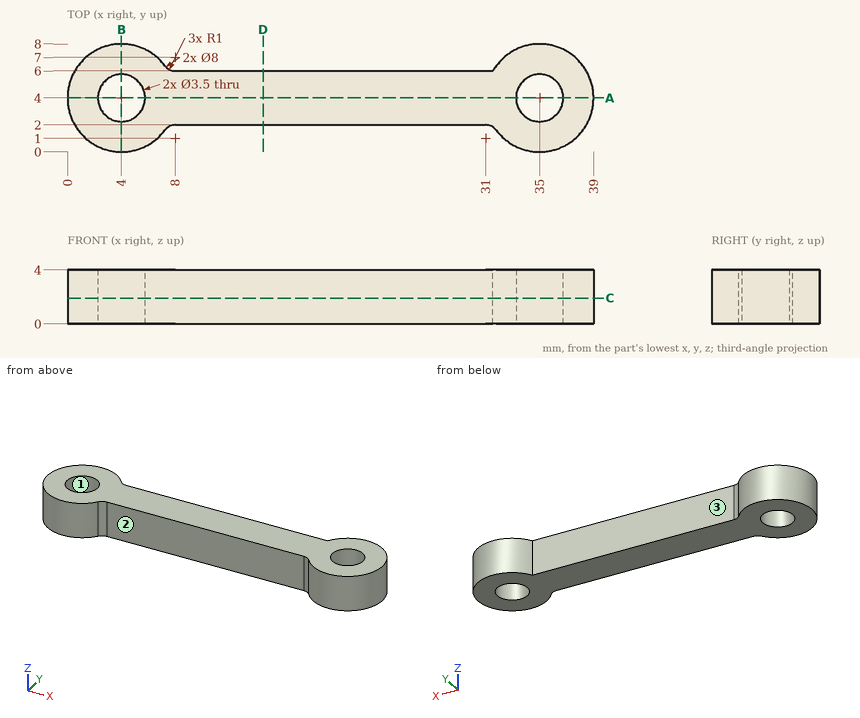
Answer from the drawing. Dimensions are ordinates in mm from the lowest x, y and z of the part. Coordinates: 2 decimals unless noted, no trailing zeros. Loops run counter-clockwise (first coordinate to the right, second up) from the corner with the lowest first, then second, coordinate; pieces in that order, holes last. Notation, with made-up numbers: (88.25, -5) - (138.25, -5) arc R11 cw to (138.25, 3) - close; hole circle Ø6 at (-34, 32). An arc over 180 degrees is marked (long way). Use a Markdown table: item, result.
Item 1: The mould has two halves that part along Y. Classify the marked faces 1, 2 and 3: +Y half, -Y half, draft (parallel to the pull), parting line (faces both ways), or undercut.
Evaluation:
| item | result |
|---|---|
| face 1 | undercut |
| face 2 | -Y half |
| face 3 | +Y half |
Item 2: Consider probe 1 along Y at (x, z) = (35, 1.9); probe 2 along X at (y, z) = (2.5, 3.15); probe 3 along X at (y, z) = (3.5, 3.85). Determine where each line is inside the solid, lowest interval first. Write a range as from..to.
Evaluation:
| item | result |
|---|---|
| probe 1 | y = 0..2.25, 5.75..8 |
| probe 2 | x = 0.29..3.1, 4.9..34.1, 35.9..38.71 |
| probe 3 | x = 0.03..2.32, 5.68..33.32, 36.68..38.97 |
Item 3: Find section A-A, the plane y = 4. Determine the outline of the cut face in (x, z).
Evaluation:
| item | result |
|---|---|
| outline | (0, 0) - (2.25, 0) - (2.25, 4) - (0, 4) - close; (5.75, 0) - (33.25, 0) - (33.25, 4) - (5.75, 4) - close; (36.75, 0) - (39, 0) - (39, 4) - (36.75, 4) - close |
Item 4: Find section B-B, the plane x = 4. Determine the outline of the cut face in (y, z), and give its area (3 significant figures).
Evaluation:
| item | result |
|---|---|
| outline | (0, 0) - (2.25, 0) - (2.25, 4) - (0, 4) - close; (5.75, 0) - (8, 0) - (8, 4) - (5.75, 4) - close |
| area | 18.0 mm2 |
Item 5: Given pin 1 Ø2 at (x, z) = (15, 1.5) entering from -Y; pin 2 Ø1.5 at (y, z) = (3, 3.5) entering from +X; pin 3 Ø3 at (x, y) = (13, 5.5) entering from -Z; pin 4 Ø1 at (y, z) = (1, 2.5) entering from -X, each flat-ended and moving along its own axis, determine where each tip first touches the part or whether it passes through.
Evaluation:
| item | result |
|---|---|
| pin 1 | stops at y = 2 |
| pin 2 | stops at x = 38.99 |
| pin 3 | stops at z = 0 |
| pin 4 | stops at x = 0.88 |
Item 6: Find section D-D, the plane x = 14.5. Determine the outline of the cut face in (y, z).
Evaluation:
| item | result |
|---|---|
| outline | (2, 0) - (6, 0) - (6, 4) - (2, 4) - close |
Item 7: Find section C-C, the plane z = 1.9. Determine the outline of the cut face in (x, y).
Evaluation:
| item | result |
|---|---|
| outline | (7.2, 1.6) arc R1 cw to (8, 2) - (31, 2) arc R1 cw to (31.8, 1.6) arc R4 ccw (long way) to (31.54, 6) - (8, 6) arc R1 cw to (7.2, 6.4) arc R4 ccw (long way) to start; hole circle Ø3.5 at (4, 4); hole circle Ø3.5 at (35, 4) |
